Autodesk Inventor part; units mm, degrees
ref_plane "YZ Plane" through (0, 0, 0) normal (1, 0, 0) x (0, 1, 0)
ref_plane "XZ Plane" through (0, 0, 0) normal (0, 1, 0) x (-1, 0, 0)
ref_plane "XY Plane" through (0, 0, 0) normal (0, 0, 1) x (1, 0, 0)
sketch "Sketch1" plane through (0, 0, 0) normal (0, 0, 1) x (1, 0, 0)
  line L0 (0, 0) -> (71, 0)
  line L1 (71, 0) -> (71, -12)
  line L2 (71, -12) -> (0, -12)
  line L3 (0, -12) -> (0, 0)
  circle A0 centre (10, -6) radius 2.1
  circle A1 centre (35.5, -6) radius 2.1
  circle A2 centre (61, -6) radius 2.1
  line L4 (71, 0) -> (51, 0)
  line L5 (51, 0) -> (51, 7.5)
  line L6 (51, 7.5) -> (71, 7.5)
  line L7 (71, 7.5) -> (71, 0)
  point P0 (0, -6)
  point P1 (71, -6)
  point P2 (35.5, 0)
  dimension "d0" = 71
  dimension "d1" = 12
  dimension "d2" = 10
  dimension "d3" = 6
  dimension "d4" = 10
  dimension "d5" = 6
  dimension "d6" = 6
  dimension "d7" = 35.5
  dimension "d8" = 4.2
  dimension "d9" = 4.2
  dimension "d10" = 4.2
  dimension "d11" = 20
  dimension "d12" = 7.5
extrude "Extrusion1" add sketch "Sketch1" along normal blind 10
equation "\"d9\" = d8"
equation "\"d10\" = d8"
properties part number "Touchscreen mount v01"
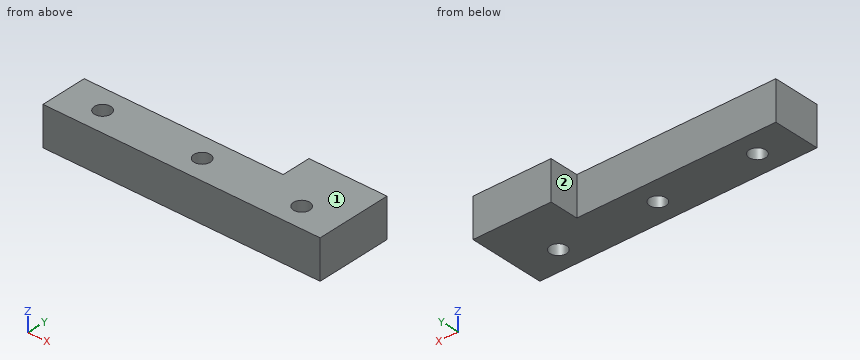
Input: part model. Units: mm. Frame: model coordinates. Face numbers are marked on the shaded views. A direction names the side the tool comes from. Round coordinates to 2 decimals unless told otherwise and drop trailing zeros. Loops run counter-clockwise (first coordinate to the right, second up) from the corner with the lowest first, then second, coordinate; pieces in that order, holes last. Notation, with made-up numbers: (-18, -15.75) -> (9, -15.75) arc R24 cw to (9, 4.25) -> close; hole circle Ø1 at (-16, 31.5). An arc over 180 degrees is marked (long way). Answer as a JSON object with one key per item and string values. Group by question number.
1) Pin query (flat end, axial travel): pin 1 (6.5 mm diameter, centred on x = 10, y = -6, fed in from -Z); pin 2 (3 mm diameter, centred on x = 21, z = 4, fed in from +Y); pin 3 (6 mm diameter, centred on y = 5.5, z = 3, fed in from -X); pin 4 (6 mm diameter, centred on x = 19.5, y = 4.5, fed in from -Z). Return the tip coordinate at first contact, or that it passes through.
2) Ray query, L1, parallel to X at y = -6.25, z = 9; L2, parallel to Y at x = 10, z = 1.25; L3, parallel to Y at x = 61, z = 5. Return the intervals inside material, ascending.
3) Reachability of the marked faces 1 and 2 from +Z, -Z, +X, -X, +Y, -Y: full face, straight path, thin tool, end or side. Return the list, or none.
4) Section query D-D on y = 4. Output: boundary loops of the cut face in (x, z), plus the area to 3 significant figures.
5) Section query C-C on x = 61. Output: boundary loops of the cut face in (y, z), plus the area to 3 significant figures.
6) Section query B-B on y = -6. Output: boundary loops of the cut face in (x, z).
7) Section query A-A on x = 10. Output: boundary loops of the cut face in (y, z), plus the area to 3 significant figures.
Reply:
{
 "1": {"pin 1": "stops at z = 0", "pin 2": "stops at y = 0", "pin 3": "stops at x = 51", "pin 4": "passes through"},
 "2": {"L1": "x = 0 to 7.91, 12.09 to 33.41, 37.59 to 58.91, 63.09 to 71", "L2": "y = -12 to -8.1, -3.9 to 0", "L3": "y = -12 to -8.1, -3.9 to 7.5"},
 "3": {"face 1": "+Z, +X, -X, +Y, -Y", "face 2": "+Z, -Z, -X, +Y"},
 "4": {"outline": "(51, 0) -> (71, 0) -> (71, 10) -> (51, 10) -> close", "area": "200 mm2"},
 "5": {"outline": "(-12, 0) -> (-8.1, 0) -> (-8.1, 10) -> (-12, 10) -> close; (-3.9, 0) -> (7.5, 0) -> (7.5, 10) -> (-3.9, 10) -> close", "area": "153 mm2"},
 "6": {"outline": "(0, 0) -> (7.9, 0) -> (7.9, 10) -> (0, 10) -> close; (12.1, 0) -> (33.4, 0) -> (33.4, 10) -> (12.1, 10) -> close; (37.6, 0) -> (58.9, 0) -> (58.9, 10) -> (37.6, 10) -> close; (63.1, 0) -> (71, 0) -> (71, 10) -> (63.1, 10) -> close"},
 "7": {"outline": "(-12, 0) -> (-8.1, 0) -> (-8.1, 10) -> (-12, 10) -> close; (-3.9, 0) -> (0, 0) -> (0, 10) -> (-3.9, 10) -> close", "area": "78.0 mm2"}
}
